Part model, mm, in its own coordinate system. A direction names the side the tool comes from. Round coordinates to 2 decimals unless told otherwise and drop trailing zeros. Order: outer loops, then holes, each group sorted by start corner. A loop starts at its lowest first (then second) coordinate and runs counter-clockwise, first axis right, second up. Notation, with made-up numbers: (-4.5, 68.25) - (5.5, 68.25) arc R8 cw to (5.5, 80.25) - close; hole circle Ø6 at (4.25, 74.25). An arc over 180 degrees is marked (long way). Answer as a JSON object with one key per item and string values.
```python
from build123d import *

# Parameters (mm, degrees)
SKETCH1_R                      = 10.16
BOSS_EXTRUDE1_DEPTH            = 6.35
SKETCH2_R                      = 11.1125
CUT_EXTRUDE1_DEPTH             = 4.7625
SKETCH3_R                      = 11.1125
SKETCH3_R_2                    = 9.8425
BOSS_EXTRUDE2_DEPTH            = 4.75996
CHAMFER1_SIZE                  = 0.254
SKETCH4_R                      = 8.5725
SKETCH4_R_2                    = 7.9375
BOSS_EXTRUDE3_DEPTH            = 4.75996
CHAMFER2_SIZE                  = 0.254
SKETCH5_R                      = 9.8425
SKETCH5_R_2                    = 8.5725
BOSS_EXTRUDE4_DEPTH            = 4.2545
F_6_32_TAPPED_HOLE1_AT_2_COUNT = 2
F_6_32_TAPPED_HOLE1_AT_2_PITCH = 26.940768363


with BuildPart() as part:
    # Sketch1 → Boss-Extrude1 (new body)
    with BuildSketch(Plane(origin=(0, 0, 0), x_dir=(1, 0, 0), z_dir=(0, 1, 0))):
        with BuildLine():
            Line((-16.764, -16.51), (-7.62, -16.51))
            Line((-7.62, -16.51), (-7.62, -14.9479))
            ThreePointArc((-7.62, -14.9479), (-7.155032015, -13.825367985), (-6.0325, -13.3604))
            Line((-6.0325, -13.3604), (6.0325, -13.3604))
            ThreePointArc((6.0325, -13.3604), (7.155032015, -13.825367985), (7.62, -14.9479))
            Line((7.62, -14.9479), (7.62, -16.51))
            Line((7.62, -16.51), (16.764, -16.51))
            Line((16.764, -16.51), (16.764, -10.4267))
            Line((16.764, -10.4267), (15.1765, -10.4267))
            ThreePointArc((15.1765, -10.4267), (14.053967985, -9.961732015), (13.589, -8.8392))
            Line((13.589, -8.8392), (13.589, 8.8392))
            ThreePointArc((13.589, 8.8392), (14.053967985, 9.961732015), (15.1765, 10.4267))
            Line((15.1765, 10.4267), (16.764, 10.4267))
            Line((16.764, 10.4267), (16.764, 16.51))
            Line((16.764, 16.51), (7.62, 16.51))
            Line((7.62, 16.51), (7.62, 14.9479))
            ThreePointArc((7.62, 14.9479), (7.155032015, 13.825367985), (6.0325, 13.3604))
            Line((6.0325, 13.3604), (-6.0325, 13.3604))
            ThreePointArc((-6.0325, 13.3604), (-7.155032015, 13.825367985), (-7.62, 14.9479))
            Line((-7.62, 14.9479), (-7.62, 16.51))
            Line((-7.62, 16.51), (-16.764, 16.51))
            Line((-16.764, 16.51), (-16.764, 10.4267))
            Line((-16.764, 10.4267), (-15.1765, 10.4267))
            ThreePointArc((-15.1765, 10.4267), (-14.053967985, 9.961732015), (-13.589, 8.8392))
            Line((-13.589, 8.8392), (-13.589, -8.8392))
            ThreePointArc((-13.589, -8.8392), (-14.053967985, -9.961732015), (-15.1765, -10.4267))
            Line((-15.1765, -10.4267), (-16.764, -10.4267))
            Line((-16.764, -10.4267), (-16.764, -16.51))
        make_face()
        Circle(SKETCH1_R, mode=Mode.SUBTRACT)
    extrude(amount=BOSS_EXTRUDE1_DEPTH)

    # Sketch2 → Cut-Extrude1 (cut)
    with BuildSketch(Plane(origin=(0, 6.35, 0), x_dir=(1, 0, 0), z_dir=(0, 1, 0))):
        Circle(SKETCH2_R)
    extrude(amount=-CUT_EXTRUDE1_DEPTH, mode=Mode.SUBTRACT)

    # Sketch3 → Boss-Extrude2 (add)
    with BuildSketch(Plane(origin=(0, 1.5875, 0), x_dir=(-1, 0, 0), z_dir=(0, 1, 0))):
        Circle(SKETCH3_R)
        Circle(SKETCH3_R_2, mode=Mode.SUBTRACT)
    extrude(amount=BOSS_EXTRUDE2_DEPTH)

    # Chamfer1
    chamfer1_edges = [part.edges().sort_by_distance(p)[0] for p in [
        (9.8425, 1.5875, 0),
        (9.8425, 6.34746, 0),
    ]]
    chamfer(chamfer1_edges, length=CHAMFER1_SIZE)



with BuildPart() as body_2:
    # Sketch4 → Boss-Extrude3 (new body)
    with BuildSketch(Plane(origin=(0, 1.5875, 0), x_dir=(-1, 0, 0), z_dir=(0, 1, 0))):
        Circle(SKETCH4_R)
        Circle(SKETCH4_R_2, mode=Mode.SUBTRACT)
    extrude(amount=BOSS_EXTRUDE3_DEPTH)

    # Chamfer2
    chamfer2_edges = [body_2.edges().sort_by_distance(p)[0] for p in [
        (8.5725, 1.5875, 0),
        (8.5725, 6.34746, 0),
    ]]
    chamfer(chamfer2_edges, length=CHAMFER2_SIZE)


with BuildPart() as part_1:
    add(part.part)

    add(body_2.part)  # Boss-Extrude4 merges body 2
    # Sketch5 → Boss-Extrude4 (add)
    with BuildSketch(Plane(origin=(0, 6.09346, 0), x_dir=(-1, 0, 0), z_dir=(0, 1, 0))):
        Circle(SKETCH5_R)
        Circle(SKETCH5_R_2, mode=Mode.SUBTRACT)
    extrude(amount=-BOSS_EXTRUDE4_DEPTH)

    # Sketch8 → #6-32 Tapped Hole1 (revolve, cut)
    with BuildSketch(Plane(origin=(-16.764, 3.175, -13.470384182), x_dir=(0, 0, 1), z_dir=(0, 1, 0))):
        Polygon((0, 0), (0, 8.76289403), (1.35255, 7.9502), (1.35255, 7.0104), (1.7526, 7.0104), (1.7526, 0), align=None)
    f_6_32_tapped_hole1 = revolve(axis=Axis((-23.114, 3.175, -13.470384182), (1, 0, 0)), mode=Mode.SUBTRACT)

    # #6-32 Tapped Hole1 at 2: #6-32 Tapped Hole1 ×2
    with Locations(*[(0, 0, i * F_6_32_TAPPED_HOLE1_AT_2_PITCH) for i in range(1, F_6_32_TAPPED_HOLE1_AT_2_COUNT)]):
        add(f_6_32_tapped_hole1, mode=Mode.SUBTRACT)

    # Mirror1: #6-32 Tapped Hole1 across plane
    add(f_6_32_tapped_hole1.mirror(Plane(origin=(0, 0, 0), x_dir=(0, 0, 1), z_dir=(1, 0, 0))), mode=Mode.SUBTRACT)

    # Mirror1 copy 1 sketch → Mirror1 copy 1 (revolve, cut)
    with BuildSketch(Plane(origin=(16.764, 3.175, 13.470384182), x_dir=(0, 0, 1), z_dir=(0, 1, 0))):
        Polygon((0, 0), (0, -8.76289403), (1.35255, -7.9502), (1.35255, -7.0104), (1.7526, -7.0104), (1.7526, 0), align=None)
    revolve(axis=Axis((23.114, 3.175, 13.470384182), (1, 0, 0)), mode=Mode.SUBTRACT)


solid = part_1.part
```
Item 1: Two-plate mould, pull along X, no slides. Class faces 1 (the flat face through (12, 3, 16.51)), 2 (the cylindrical face through (-14.04, 3.13, 9.95)), 3 (the cylindrical face through (-7.14, 3.13, -13.81)): pulls with the +X half, pulls with the -X half, needs draft (parallel to the pull), parting line crosses it, or undercut.
Taken from the geometry:
{"face 1": "needs draft", "face 2": "pulls with the -X half", "face 3": "undercut"}
Item 2: Cut at B-B (x = -12). Write the cut outline in (y, z) (3 decimals).
Taken from the geometry:
{"outline": "(0, -16.51) - (6.35, -16.51) - (6.35, 16.51) - (0, 16.51) - close; hole circle Ø3.505 at (3.175, -13.47); hole circle Ø3.505 at (3.175, 13.47)"}
Item 3: Probe L1, parallel to Z at x = -15, y = 1; L2, parallel to X at y = 6.25, z = 5.5; L3, parallel to X at y = 0.95, z = 0. List the from-to ranges inside material, lowest first. Write a range as from..to.
Taken from the geometry:
{"L1": "-16.51..-10.42, 10.42..16.51", "L2": "-13.59..-8.35, -6.37..-5.72, 5.72..6.37, 8.35..13.59", "L3": "-13.59..-10.16, 10.16..13.59"}
Item 4: Drop flat-ended pins along their axis: P1, Ø19.5, axis at x = 0, z = 0, coming from the +Y side; P2, Ø2, axis at y = 3.18, z = -13.47, coming from the -X side (3 decimals); P3, Ø8.5, axis at x = -2.5, z = 3, coming from the -Y side. Give the stop position or say it passes through.
Taken from the geometry:
{"P1": "y = 6.35", "P2": "x = -8.605", "P3": "y = 1.59"}
Item 5: Cut at A-A (x = 14). Write the cut outline in (y, z) (3 decimals), plus the area to 3 significant figures.
Taken from the geometry:
{"outline": "(0, -16.51) - (6.35, -16.51) - (6.35, -9.905) - (0, -9.905) - close; (0, 9.905) - (6.35, 9.905) - (6.35, 16.51) - (0, 16.51) - close; hole circle Ø3.505 at (3.175, -13.47); hole circle Ø3.505 at (3.175, 13.47)", "area": "64.6 mm2"}
Item 6: Tool access for faces 4 (the cylindrical face through (14.066, 3.131, 9.974)), 5 (the cylindrical face through (-9.29, 3.69, -12.22)), 6 (the flat face through (-1, 6.093, 9)), 7 (the flat face through (-1, 1.839, 9)), 8 (the cylindrical face through (13.308, 2.649, 15.142)): list every direction of +Z, -Z, +X, -X, +Y, -Y with a clear straight run to the whole face (end or side of a thin tool).
Taken from the geometry:
{"face 4": "+X, +Y, -Y", "face 5": "-X", "face 6": "+Y", "face 7": "-Y", "face 8": "+X"}
